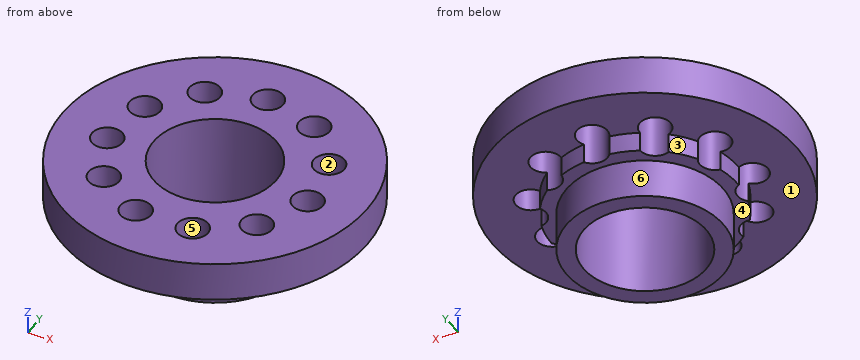
from build123d import *

# Parameters (mm, degrees)
F0_R     = 4
F0_R_2   = 3.125
F1_DEPTH = 5
F2_R     = 7.75
F2_R_2   = 4
F3_DEPTH = 2
F4_R     = 4.75
F4_R_2   = 4
F5_DEPTH = 1
F6_R     = 0.7799623088
F7_DEPTH = 12.7


with BuildPart() as f1:
    # F0 (on Top) → F1 (new body)
    with BuildSketch(Plane.XY):
        Circle(F0_R)
        Circle(F0_R_2, mode=Mode.SUBTRACT)
    extrude(amount=F1_DEPTH)

    # F2 (on face) → F3 (join)
    with BuildSketch(Plane.XY.offset(5)):
        Circle(F2_R)
        Circle(F2_R_2, mode=Mode.SUBTRACT)
    extrude(amount=-F3_DEPTH)

    # F4 (on face) → F5 (join)
    with BuildSketch(Plane(origin=(0, 0, 3), x_dir=(1, 0, 0), z_dir=(0, 0, -1))):
        Circle(F4_R)
        Circle(F4_R_2, mode=Mode.SUBTRACT)
    extrude(amount=F5_DEPTH)

    # F6 (on face) → F7 (cut, symmetric)
    with BuildSketch(Plane.XY.offset(5)):
        with Locations((0, 5.1454929635)):
            Circle(F6_R)
        with Locations((-2.781863522, 4.3286641337)):
            Circle(F6_R)
        with Locations((-4.6805050315, 2.1375150263)):
            Circle(F6_R)
        with Locations((-5.0931192643, -0.7322799989)):
            Circle(F6_R)
        with Locations((-3.888704117, -3.3695812986)):
            Circle(F6_R)
        with Locations((-1.4496528888, -4.9370643443)):
            Circle(F6_R)
        with Locations((1.4496528888, -4.9370643443)):
            Circle(F6_R)
        with Locations((3.888704117, -3.3695812986)):
            Circle(F6_R)
        with Locations((5.0931192643, -0.7322799989)):
            Circle(F6_R)
        with Locations((4.6805050315, 2.1375150263)):
            Circle(F6_R)
        with Locations((2.781863522, 4.3286641337)):
            Circle(F6_R)
    extrude(amount=F7_DEPTH, both=True, mode=Mode.SUBTRACT)


solid = f1.part
Input: part model. Units: mm. Frame: model coordinates. Face numbers are marked on the shaded views. A direction names the side the tool comes from. Give positions to 0.01 mm unless a question says otherwise; leave off trailing zeros. Loops run counter-clockwise (first coordinate to the right, second up) from the corner with the lowest first, then second, coordinate; pieces in that order, holes last. Notation, with made-up numbers: (-12, -27) -> (-8, -27) arc R27 cw to (-8, 10) -> close; hole circle Ø2 at (-15.75, 76). An arc over 180 degrees is marked (long way). Answer as a JSON object with one key per item and string values. Group by question number.
Item 1: Line query: probe 1 along X at (y, z) = (-1, 3.5); probe 2 along X at (y, z) = (-4.25, 4.1); probe 3 along X at (y, z) = (3.75, 4). Output: solid intervals per line, ascending.
Item 2: Cut plane A-A, the plane y = 1.75. Return the cut outline in (x, z), and give its area (3 significant figures).
Item 3: Pin query (flat end, axial travel): P1, Ø1.4, axis at x = -1.45, y = -4.94, coming from the -Z side; P2, Ø2, axis at x = 6, z = 3.5, coming from the +Y side; P3, Ø2, axis at x = -4.68, y = 2.14, coming from the -Z side; P4, Ø3, axis at x = -5, y = 6, coming from the -Z side. Return the tip coordinate at first contact, or that it passes through.
Item 4: Reachability of the marked faces 1, 2 and 3 from +Z, -Z, +X, -X, +Y, -Y: full face, straight path, thin tool, end or side. Return the list, or none.
Item 5: Cut plane C-C, the plane z = 0.7. Return the cut outline in (x, y) (3 decimals), and give its area (3 significant figures).
Item 6: Pull-direction query (Y, two-part tool) for the marked faces 4, 5 and 6; classes: released by +Y, released by -Y, zero draft, split by the parting line, or undercut.
Item 7: Cut plane B-B, the plane x = 0. Return the cut outline in (y, z) (3 decimals), and give its area (3 significant figures).
Item 8: Cut plane D-D, the plane y = -2.25. Return the cut outline in (x, z), and give its area (3 significant figures).
Checks:
{
 "1": {"probe 1": "x = -7.69 to -5.83, -4.36 to -2.96, 2.96 to 4.36, 5.83 to 7.69", "probe 2": "x = -6.48 to -1.82, -1.08 to 1.08, 1.82 to 6.48", "probe 3": "x = -6.78 to -3.3, -2.26 to 2.26, 3.3 to 6.78"},
 "2": {"outline": "(-7.55, 3) -> (-5.36, 3) -> (-5.36, 5) -> (-7.55, 5) -> close; (-4, 2) -> (-3.6, 2) -> (-3.6, 0) -> (-2.59, 0) -> (-2.59, 5) -> (-4, 5) -> close; (2.59, 0) -> (3.6, 0) -> (3.6, 2) -> (4, 2) -> (4, 5) -> (2.59, 5) -> close; (5.36, 3) -> (7.55, 3) -> (7.55, 5) -> (5.36, 5) -> close", "area": "21.3 mm²"},
 "3": {"P1": "passes through", "P2": "stops at y = 5.92", "P3": "stops at z = 2", "P4": "stops at z = 3"},
 "4": {"face 1": "-Z", "face 2": "+Z, -Z", "face 3": "-Z, -X, +Y"},
 "5": {"outline": "circle Ø8 at (0, 0); hole circle Ø6.25 at (0, 0)", "area": "19.6 mm²"},
 "6": {"face 4": "zero draft", "face 5": "undercut", "face 6": "split by the parting line"},
 "7": {"outline": "(-7.75, 3) -> (-4.75, 3) -> (-4.75, 2) -> (-4, 2) -> (-4, 0) -> (-3.125, 0) -> (-3.125, 5) -> (-7.75, 5) -> close; (3.125, 0) -> (4, 0) -> (4, 2) -> (4.366, 2) -> (4.366, 5) -> (3.125, 5) -> close; (5.925, 3) -> (7.75, 3) -> (7.75, 5) -> (5.925, 5) -> close", "area": "21.7 mm²"},
 "8": {"outline": "(-7.42, 3) -> (-4.18, 3) -> (-4.18, 2) -> (-3.31, 2) -> (-3.31, 0) -> (-2.17, 0) -> (-2.17, 5) -> (-7.42, 5) -> close; (2.17, 0) -> (3.31, 0) -> (3.31, 2) -> (4.18, 2) -> (4.18, 3) -> (7.42, 3) -> (7.42, 5) -> (2.17, 5) -> close", "area": "29.6 mm²"}
}
